Part print with two shaded views. Sizes in mm from the minimum x, y, z corner. A direction names the side the tool comes from. Round coordinates to 2 decimals unless told otherwise and drop trailing zeros. Loops run counter-clockwise (first coordinate to the right, second up) from the corner with the lowest first, then second, coordinate; pieces in that order, holes last. Notation, with made-up numbers: (84.5, 89.25) - (106.5, 89.25) arc R19 cw to (106.5, 98.25) - close; hole circle Ø8 at (21.25, 19.25). An arc over 180 degrees is marked (long way). One line per question, with ' | ' between items.
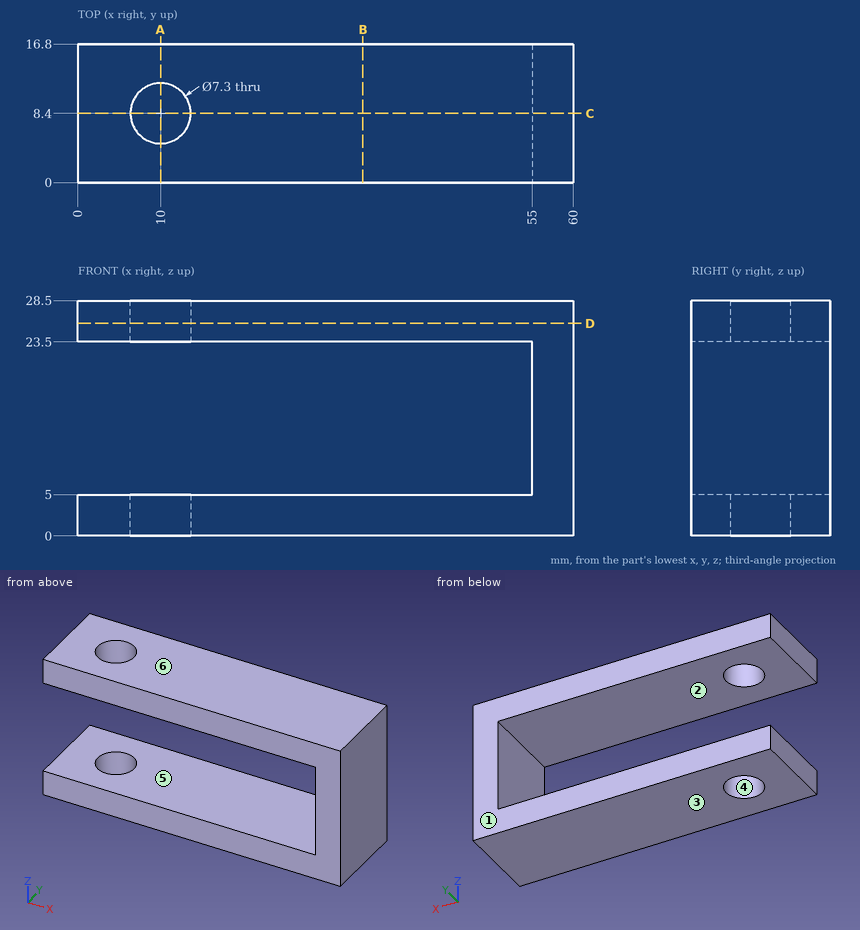
(1) Cut at A-A, the plane x = 10. Write the cut outline in (y, z), then the cut area to 3 significant figures.
Results found:
outline: (0, 0) - (4.75, 0) - (4.75, 5) - (0, 5) - close; (0, 23.5) - (4.75, 23.5) - (4.75, 28.5) - (0, 28.5) - close; (12.05, 0) - (16.8, 0) - (16.8, 5) - (12.05, 5) - close; (12.05, 23.5) - (16.8, 23.5) - (16.8, 28.5) - (12.05, 28.5) - close | area: 95.0 mm²
(2) Cut at C-C, the plane y = 8.4. Write the cut outline in (x, z).
Results found:
outline: (0, 0) - (6.35, 0) - (6.35, 5) - (0, 5) - close; (0, 23.5) - (6.35, 23.5) - (6.35, 28.5) - (0, 28.5) - close; (13.65, 0) - (60, 0) - (60, 28.5) - (13.65, 28.5) - (13.65, 23.5) - (55, 23.5) - (55, 5) - (13.65, 5) - close
(3) Drop a flat-ended pin along its axis: P1, Ø6, axis at x = 19.5, z = 18, coming from the +Y side. Give the stop position or say it passes through.
Results found:
P1: passes through
(4) Cut at D-D, the plane z = 25.75. Write the cut outline in (x, y), then the cut area to 3 significant figures.
Results found:
outline: (0, 0) - (60, 0) - (60, 16.8) - (0, 16.8) - close; hole circle Ø7.3 at (10, 8.4) | area: 966 mm²
(5) Two-plate mould, pull along Z, no slides. Class the marked faces 3, 4, 5 and 6: released by +Z, released by -Z, zero draft, split by the parting line, or undercut.
Results found:
face 3: released by -Z | face 4: zero draft | face 5: undercut | face 6: released by +Z
(6) Probe L1, parallel to Y at x = 10, z = 3.75; L2, parallel to Z at x = 14, y = 6.5; L3, parallel to X at y = 13.5, z = 18. List the from-to ranges inside material, lowest first.
Results found:
L1: y = 0 to 4.75, 12.05 to 16.8 | L2: z = 0 to 5, 23.5 to 28.5 | L3: x = 55 to 60
(7) Tool access for the marked faces 1 and 2: list every direction of +Z, -Z, +X, -X, +Y, -Y with a clear straight run to the whole face (end or side of a thin tool).
Results found:
face 1: +Z, -Z, +X, -X, +Y | face 2: -X, +Y, -Y
(8) Cut at B-B, the plane x = 34.5. Write the cut outline in (y, z).
Results found:
outline: (0, 0) - (16.8, 0) - (16.8, 5) - (0, 5) - close; (0, 23.5) - (16.8, 23.5) - (16.8, 28.5) - (0, 28.5) - close
